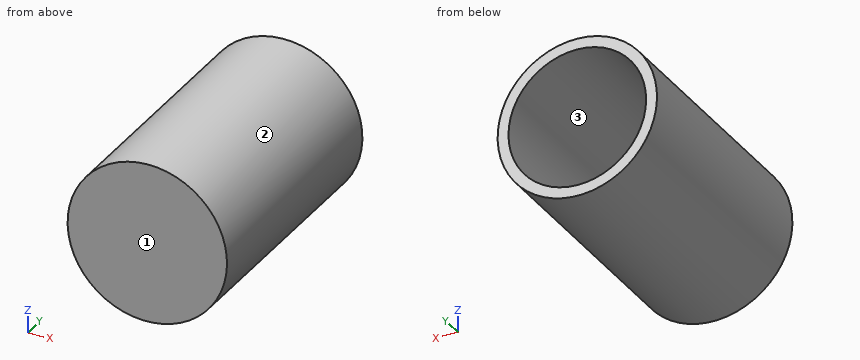
```python
from build123d import *

# Parameters (mm, degrees)
SKETCH1_R                       = 18.35
BOSS_EXTRUDE1_DEPTH             = 59.1
SKETCH2_R                       = 15.85
CUT_EXTRUDE1_DEPTH              = 57.1
BOSS_EXTRUDE2_REACH             = 66.547
BOSS_EXTRUDE2_DIRECTION_2_REACH = 66.547


with BuildPart() as part:
    # Sketch1 → Boss-Extrude1 (new body)
    with BuildSketch(Plane(origin=(0, 0, 0), x_dir=(1, 0, 0), z_dir=(0, 1, 0))):
        with Locations(Location((0, 0, 0), (0, 0, 270))):
            Circle(SKETCH1_R)
    extrude(amount=BOSS_EXTRUDE1_DEPTH)

    # Sketch2 → Cut-Extrude1 (cut)
    with BuildSketch(Plane(origin=(0, 59.1, 0), x_dir=(1, 0, 0), z_dir=(0, 1, 0))):
        with Locations(Location((0, 0, 0), (0, 0, 270))):
            Circle(SKETCH2_R)
    extrude(amount=-CUT_EXTRUDE1_DEPTH, mode=Mode.SUBTRACT)

    # Sketch3 → Boss-Extrude2 (add, up to next)
    with BuildSketch(Plane.XY, mode=Mode.PRIVATE) as boss_extrude2_sk1:
        Polygon((-15.85, 33.7), (15.85, 2), (-15.85, 2), align=None)
    boss_extrude2_tool1 = extrude(boss_extrude2_sk1.sketch, amount=BOSS_EXTRUDE2_REACH, mode=Mode.PRIVATE) - part.part
    add(boss_extrude2_tool1.solids().sort_by_distance((-5.283333, 12.566667, 0))[0])

    # Sketch3 → Boss-Extrude2 direction 2 (add, up to next)
    with BuildSketch(Plane.XY, mode=Mode.PRIVATE) as boss_extrude2_direction_2_sk1:
        Polygon((-15.85, 33.7), (15.85, 2), (-15.85, 2), align=None)
    boss_extrude2_direction_2_tool1 = extrude(boss_extrude2_direction_2_sk1.sketch, amount=-BOSS_EXTRUDE2_DIRECTION_2_REACH, mode=Mode.PRIVATE) - part.part
    add(boss_extrude2_direction_2_tool1.solids().sort_by_distance((-5.283333, 12.566667, 0))[0])


solid = part.part
```
CAD build for the part. Positions are in the model's coordinates, mm. Face numbers are marked on the shaded views. Round coordinates to 2 decimals unless told otherwise and drop trailing zeros. Loops run counter-clockwise (first coordinate to the right, second up) from the corner with the lowest first, then second, coordinate; pieces in that order, holes last. Notation, with made-up numbers: M 20,19.25 L 31,19.25 A19 ccw 31,27.25 Z; hole C 4,74 d5. An arc over 180 degrees is marked long. Use a Markdown table: item, result. Add a question column.
(1) Cut at C-C (y = 43.5). Give the cut face in (x, z).
(2) Flat gauge pins, fed straight in: pin 1 (2 mm diameter, centred on y = 48, z = 8.5, fed in from +X); pin 2 (12 mm diameter, centred on x = -11, y = 44.5, fed in from +Z); pin 3 (8 mm diameter, centred on x = 10, y = 47, fed in from -Z). Where does each tip first touch, or does it go through?
(3) Cut at B-B (x = -9.5). Give the cut face in (y, z), and give its area (3 significant figures).
(4) Cut at D-D (y = 16). Give the cut face in (x, z).
(5) Pull direction Z, two halves, no side cores. Call the marked faces 1, 2 and 3: +Z half, -Z half, draft (parallel to the pull), parting line (faces both ways), or undercut.
(6) Cut at A-A (z = -4.5). Give the cut face in (x, y), and give its area (3 significant figures).
(7) Drill centre lines: line 1 (X direction, y = 38.5, z = -6.5); line 2 (X direction, y = 50.5, z = -4); line 3 (Z direction, x = 6, y = 39). Where is each one in solid material? Low to high.
Geometry says:
| question | item | result |
|---|---|---|
| 1 | outline | C 0,0 d36.7; hole C 0,0 d31.7 |
| 2 | pin 1 | stops at x = 16.75 |
| 2 | pin 2 | stops at z = 17.66 |
| 2 | pin 3 | stops at z = -17.34 |
| 3 | outline | M 0,-15.7 L 59.1,-15.7 L 59.1,-12.69 L 27.35,-12.69 L 27.35,12.69 L 59.1,12.69 L 59.1,15.7 L 0,15.7 Z |
| 3 | area | 1,050 mm² |
| 4 | outline | C 0,0 d36.7; hole M 1.85,-15.74 A15.85 ccw 1.85,15.74 Z |
| 5 | face 1 | draft |
| 5 | face 2 | parting line |
| 5 | face 3 | undercut |
| 6 | outline | M -17.79,0 L 17.79,0 L 17.79,59.1 L 15.2,59.1 L 15.2,2.65 L -15.2,33.05 L -15.2,59.1 L -17.79,59.1 Z |
| 6 | area | 849 mm² |
| 7 | line 1 | x = -17.16 to -14.46, 14.46 to 17.16 |
| 7 | line 2 | x = -17.91 to -15.34, 15.34 to 17.91 |
| 7 | line 3 | z = -17.34 to -14.67, 14.67 to 17.34 |
